from build123d import *

# Parameters (mm, degrees)
F0_R     = 3.175
F1_DEPTH = 3.175


with BuildPart() as f1:
    # F0 (on Front) → F1 (new body, symmetric)
    with BuildSketch(Plane.XZ):
        with BuildLine():
            ThreePointArc((6.35, -1e-06), (0, 6.35), (-6.35, -1e-06))
            Line((-6.35, -1e-06), (-6.35, -95.25))
            ThreePointArc((-6.35, -95.25), (0, -101.6), (6.35, -95.25))
            Line((6.35, -95.25), (6.35, -1e-06))
        make_face()
        with Locations((0, -95.25)):
            Circle(F0_R, mode=Mode.SUBTRACT)
        Circle(F0_R, mode=Mode.SUBTRACT)
    extrude(amount=F1_DEPTH, both=True)


solid = f1.part
Check sheet for the modelled part. Datum: model origin and axes. Units: mm. Give positions to 0.01 mm unless a question says otherwise; leave off trailing zeros. Order: outer loops, then holes, each group sorted by start corner. A loop starts at its lowest first (then second) coordinate and runs counter-clockwise, first axis right, second up. Notation, with made-up numbers: M 27.25,-3.5 L 46.25,-3.5 A16 ccw 46.25,7.5 Z; hole C 50,-31.5 d1. An arc over 180 degrees is marked long. Answer as CSV lines item,"result". Start each with the question number.
Item 1: Thickness scan on line 1 (Z direction, x = 0, y = 1.5) (3 decimals); line 2 (Z direction, x = -1.5, y = 0); line 3 (Z direction, x = 5.5, y = 0.5). Record the ranges inside material, lowest first. Write a range as [from, to].
Item 2: Mould release check, pull along Z, two halves, no side actions. Record for faces 1 (the face through (-0.4, 0, -92.1)), 2 (the face through (0.14, -0.04, 6.35)), 3 (the face through (0, 3.175, -47)): +Z half, -Z half, draft (parallel to the pull), parting line (faces both ways), or undercut.
Item 3: Gauge pin test, flat ends, axial feed: P1, Ø2, axis at x = -2.5, y = 1, coming from the +Z side; P2, Ø1, axis at x = 4.5, y = 2.5, coming from the +Z side; P3, Ø3, axis at x = -3.5, y = 1.5, coming from the +Z side. Record the tip position at first contact, or that the pin passes through.
Item 4: Cross-section at A-A on x = 0. Enter the section's corners in (y, z) (3 decimals).
Item 5: Cross-section at B-B on y = -2.25. Enter the section's corners in (x, z) (3 decimals).
Established:
1,line 1,"z = [-101.6, -98.425], [-92.075, -3.175], [3.175, 6.35]"
1,line 2,"z = [-101.42, -98.05], [-92.45, -2.8], [2.8, 6.17]"
1,line 3,"z = [-98.42, 3.17]"
2,face 1,"undercut"
2,face 2,"+Z half"
2,face 3,"draft"
3,P1,"stops at z = 6.17"
3,P2,"stops at z = 4.93"
3,P3,"stops at z = 6.03"
4,outline,"M -3.175,-101.6 L 3.175,-101.6 L 3.175,-98.425 L -3.175,-98.425 Z; M -3.175,-92.075 L 3.175,-92.075 L 3.175,-3.175 L -3.175,-3.175 Z; M -3.175,3.175 L 3.175,3.175 L 3.175,6.35 L -3.175,6.35 Z"
5,outline,"M -6.35,-95.25 A6.35 ccw 6.35,-95.25 L 6.35,0 A6.35 ccw -6.35,0 Z; hole C 0,-95.25 d6.35; hole C 0,0 d6.35"
